Source: CAD feature listing. Evaluate the final solid. Frame: model axes, mm. A direction names the side the tool comes from. Give positions to 0.01 mm unless a question says otherwise; leave off trailing zeros. Order: outer loops, then holes, each group sorted by start corner. A loop starts at its lowest first (then second) coordinate and runs counter-clockwise, first axis right, second up. Notation, with made-up numbers: (6, 59) - (39, 59) arc R30 ccw to (39, 98) - close; hole circle Ø9 at (71.5, 63.25). An arc over 180 degrees is marked (long way). Use CSV: the item, a comma, the result in double quotes.
```python
from build123d import *

# Parameters (mm, degrees)
F1_DEPTH     = 20
F2_DEPTH     = 40
F3_T4_DEPTH  = 108
F3_T9_DEPTH  = 108
F3_T11_DEPTH = 76
F3_T13_DEPTH = 66
F4_R         = 10
F5_DEPTH     = 25
F6_R         = 4
F7_DEPTH     = 16
F8_DEPTH     = 25


# Not quite as in the source:
# - a fillet or chamfer that OpenCascade refuses, or shapes differently, is made with other operations: its cross-section is extruded or revolved along the edge and cut away or added


with BuildPart() as f1:
    # F0 (on Right) → F1 (new body, symmetric)
    with BuildSketch(Plane.YZ):
        with BuildLine():
            Line((40.2060094365, 37.9128916849), (0, 26))
            Line((0, 26), (108, 26))
            Line((108, 26), (108, 58))
            Line((108, 58), (64.1759622542, 45.0150999272))
            ThreePointArc((64.1759622542, 45.0150999272), (60.3700612912, 45.4148233324), (57.9615300422, 48.3886488422))
            Line((57.9615300422, 48.3886488422), (43.5795583515, 44.1273238969))
            ThreePointArc((43.5795583515, 44.1273238969), (43.1798349463, 40.3214229339), (40.2060094365, 37.9128916849))
        make_face()
    extrude(amount=F1_DEPTH, both=True)

    # F0 (on Right) → F2 (join, symmetric)
    with BuildSketch(Plane.YZ):
        Polygon((0, 26), (0, 0), (24, 0), (24, 10), (108, 10), (108, 26), align=None)
    extrude(amount=F2_DEPTH, both=True)

    # F3: fillet of radius 10 on 6 edges, made by hand


with BuildPart() as f3_tool2:
    # F3_s3 → F3_t4 (new body)
    with BuildSketch(Plane.XZ):
        with BuildLine():
            ThreePointArc((30, 26), (22.9289321881, 28.9289321881), (20, 36))
            Line((20, 36), (20, 26))
            Line((20, 26), (30, 26))
        make_face()
    extrude(amount=-F3_T4_DEPTH)

    split(bisect_by=Plane(origin=(0, -7.0819672131, 23.9016393443), x_dir=(1, 0, 0), z_dir=(0, 0.2840883297, -0.9587981127)), keep=Keep.TOP)


with BuildPart() as f1_1:
    add(f1.part)

    # F3_t1: union F3_tool2
    add(f3_tool2.part)


with BuildPart() as f3_tool7:
    # F3_s8 → F3_t9 (new body)
    with BuildSketch(Plane.XZ):
        with BuildLine():
            ThreePointArc((-30, 26), (-22.9289321881, 28.9289321881), (-20, 36))
            Line((-20, 36), (-20, 26))
            Line((-20, 26), (-30, 26))
        make_face()
    extrude(amount=-F3_T9_DEPTH)

    split(bisect_by=Plane(origin=(0, -7.0819672131, 23.9016393443), x_dir=(1, 0, 0), z_dir=(0, 0.2840883297, -0.9587981127)), keep=Keep.TOP)


with BuildPart() as f1_2:
    add(f1_1.part)

    # F3_t6: union F3_tool7
    add(f3_tool7.part)

    # F3_s12 → F3_t11 (cut)
    with BuildSketch(Plane.XY.offset(-25)):
        with BuildLine():
            ThreePointArc((30, 0), (37.0710678119, 2.9289321881), (40, 10))
            Line((40, 10), (40, 0))
            Line((40, 0), (30, 0))
        make_face()
        with BuildLine():
            ThreePointArc((-30, 0), (-37.0710678119, 2.9289321881), (-40, 10))
            Line((-40, 10), (-40, 0))
            Line((-40, 0), (-30, 0))
        make_face()
    extrude(amount=F3_T11_DEPTH, mode=Mode.SUBTRACT)

    # F3_s14 → F3_t13 (cut)
    with BuildSketch(Plane.XY.offset(-15)):
        with BuildLine():
            ThreePointArc((30, 108), (37.0710678119, 105.0710678119), (40, 98))
            Line((40, 98), (40, 108))
            Line((40, 108), (30, 108))
        make_face()
        with BuildLine():
            ThreePointArc((-30, 108), (-37.0710678119, 105.0710678119), (-40, 98))
            Line((-40, 98), (-40, 108))
            Line((-40, 108), (-30, 108))
        make_face()
    extrude(amount=F3_T13_DEPTH, mode=Mode.SUBTRACT)

    # F4 (on face) → F5 (cut)
    with BuildSketch(Plane(origin=(0, -7.0819672131, 23.9016393443), x_dir=(1, 0, 0), z_dir=(0, -0.2840883297, 0.9587981127))):
        with Locations((0, 95.0273192946)):
            Circle(F4_R)
    extrude(amount=-F5_DEPTH, mode=Mode.SUBTRACT)

    # F6 (on face) → F7 (cut, through all)
    with BuildSketch(Plane.XY.offset(26)):
        with Locations((30, 40)):
            Circle(F6_R)
        with Locations((-30, 40)):
            Circle(F6_R)
    extrude(amount=-F7_DEPTH, mode=Mode.SUBTRACT)

    # F6 (on face) → F8 (cut)
    with BuildSketch(Plane.XY.offset(26)):
        with Locations((30, 40)):
            Circle(F6_R)
        with Locations((-30, 40)):
            Circle(F6_R)
    extrude(amount=F8_DEPTH, mode=Mode.SUBTRACT)


solid = f1_2.part
```
Item 1: Set-up query: faces 1 (the flat face through (1, 24, 5)), 2 (the flat face through (35, 55, 26)), 3 (the flat face through (-20, 79, 42)). Return all of +Z, -Z, +X, -X, +Y, -Y with unobstructed straight access to the full face (end or side cutting, diameter ignored); none if empty.
Filled in:
face 1,"-Z, +X, -X, +Y"
face 2,"+Z, +X, +Y, -Y"
face 3,"+Z, -X, +Y, -Y"
Item 2: First-contact query: pin 1 (10 mm diameter, centred on x = 5, y = 51.5, fed in from +Z); pin 2 (2 mm diameter, centred on x = -1, y = 61.5, fed in from +Z); pin 3 (4 mm diameter, centred on x = 5, y = 34, fed in from +Z). Flat tips, straight axial feed; report the tip coordinate or a pass-through.
Filled in:
pin 1,"stops at z = 47.96"
pin 2,"stops at z = 45.35"
pin 3,"stops at z = 36.67"
Item 3: Section A-A on x = 12. Return the cut outline in (y, z).
Filled in:
outline,"(0, 0) - (24, 0) - (24, 10) - (108, 10) - (108, 58) - (64.18, 45.02) arc R5 cw to (57.96, 48.39) - (43.58, 44.13) arc R5 cw to (40.21, 37.91) - (0, 26) - close"
Item 4: Material intervals for line 1 (Y direction, x = -30, z = 18); line 2 (X direction, y = 40, z = 15); line 3 (Z direction, x = 30, y = 56), sorted ascending. Write a range as from..to.
Filled in:
line 1,"y = 0..36, 44..108"
line 2,"x = -40..-34, -26..26, 34..40"
line 3,"z = 10..26"
Item 5: Section C-C on x = -2.5. Return the cut outline in (y, z), then the cut area to 3 significant figures.
Filled in:
outline,"(0, 0) - (24, 0) - (24, 10) - (108, 10) - (108, 58) - (93.31, 53.65) - (100.42, 29.68) - (81.85, 24.18) - (74.75, 48.15) - (64.18, 45.02) arc R5 cw to (57.96, 48.39) - (43.58, 44.13) arc R5 cw to (40.21, 37.91) - (0, 26) - close"
area,"3,300 mm2"
Item 6: Mould query, pull axis Z, two halves, no side actions, for faces 4 (the cylindrical face through (-36.99, 105.15, 17.89)), 5 (the cylindrical face through (23.01, 65.24, 28.85)), 6 (the cylindrical face through (-1.302, 97.038, 41.897)). Classes: released by +Z, released by -Z, zero draft, split by the parting line, or undercut.
Filled in:
face 4,"zero draft"
face 5,"released by +Z"
face 6,"undercut"
Item 7: Section B-B on y = 49. Return the cut outline in (x, z).
Filled in:
outline,"(-40, 10) - (40, 10) - (40, 26) - (30, 26) arc R10 cw to (20, 36) - (20, 45.73) - (-20, 45.73) - (-20, 36) arc R10 cw to (-30, 26) - (-40, 26) - close"
